Build history of the part. All positions in model axes, mm. A direction names the side the tool comes from. Give positions to 0.01 mm unless a question says otherwise; leave off trailing zeros. Order: outer loops, then holes, each group sorted by start corner. A loop starts at its lowest first (then second) coordinate and runs counter-clockwise, first axis right, second up. Notation, with made-up numbers: M 60.5,1 L 65.5,1 A32 cw 65.5,30 Z; hole C 18.25,52.25 d10. An arc over 180 degrees is marked long. Use CSV: the item, a comma, the result in double quotes. Start each with the question number.
Item 1: Two-plate mould, pull along X, no slides. Class faces 1 (the flat face through (-15, 25.4, -15)), 2 (the cylindrical face through (-26.13, 16.74, -4.58)), 3 (the flat face through (-18, 36.83, -17)): pulls with the +X half, pulls with the -X half, needs draft (parallel to the pull), parting line crosses it, or undercut.
Item 2: Pin check, flat tips, straight feed: P1, Ø4, axis at x = -26.5, y = 17.5, coming from the +Z side; P2, Ø10, axis at x = -8.5, z = -25, coming from the -Y side; P3, Ø4, axis at x = -11.5, y = 37, coming from the +Z side; P4, Ø6.5, axis at x = -17, z = -12, coming from the -Y side. Stop position of each tip, or through.
Item 3: Which spindle directions (+Z, -Z, +X, -X, +Y, -Y) get a long thin tool onto all of the face, cutting with end or side? Do faces 4 (the cylindrical face through (-25.84, 12.52, -12.89)), 5 (the cylindrical face through (-17.343, 40.587, -12.947)), 6 (the cylindrical face through (-4.58, 16.74, -4.35)). Say none if no direction does.
Item 4: Band-saw the part on D-D on x = -16. Write the cut outline in (y, z), plus the area to 3 significant figures.
Item 5: Wall check: line 1 along X through (y, z) = (5, -15); line 2 along Y through (x, z) = (-6.5, -21.5). Give the ranges that are in metal, low to high.
Item 6: Band-saw the part on C-C on z = -6.5. Write the cut outline in (x, y), plus the area to 3 significant figures.
from build123d import *

# Parameters (mm, degrees)
SKETCH3_W           = 30.48
SKETCH3_H           = 30.48
BOSS_EXTRUDE1_DEPTH = 33.02
SKETCH4_R           = 5.08
BOSS_EXTRUDE2_DEPTH = 3.81
SKETCH5_R           = 3.1115
BOSS_EXTRUDE3_DEPTH = 7.62
SKETCH6_R           = 10.8585
CUT_EXTRUDE1_DEPTH  = 25.4
FILLET1_R           = 15.24


with BuildPart() as part:
    # Sketch3 → Boss-Extrude1 (new body)
    with BuildSketch(Plane(origin=(0, 0, 0), x_dir=(1, 0, 0), z_dir=(0, 1, 0))):
        with Locations((-15.24, 15.24)):
            Rectangle(SKETCH3_W, SKETCH3_H)
    extrude(amount=BOSS_EXTRUDE1_DEPTH)

    # Sketch4 → Boss-Extrude2 (add)
    with BuildSketch(Plane(origin=(0, 33.02, 0), x_dir=(1, 0, 0), z_dir=(0, 1, 0))):
        with Locations(Location((-15.24, 15.24, 0), (0, 0, 90))):
            Circle(SKETCH4_R)
    extrude(amount=BOSS_EXTRUDE2_DEPTH)

    # Sketch5 → Boss-Extrude3 (add)
    with BuildSketch(Plane(origin=(0, 36.83, 0), x_dir=(1, 0, 0), z_dir=(0, 1, 0))):
        with Locations(Location((-15.24, 15.24, 0), (0, 0, 90))):
            Circle(SKETCH5_R)
    extrude(amount=BOSS_EXTRUDE3_DEPTH)

    # Sketch6 → Cut-Extrude1 (cut)
    with BuildSketch(Plane.XZ):
        with Locations(Location((-15.24, -15.24, 0), (0, 0, 270))):
            Circle(SKETCH6_R)
    extrude(amount=-CUT_EXTRUDE1_DEPTH, mode=Mode.SUBTRACT)

    # Fillet1
    fillet1_edges = [part.edges().sort_by_distance(p)[0] for p in [
        (-30.48, 16.51, -30.48),
        (0, 16.51, -30.48),
        (-30.48, 16.51, 0),
        (0, 16.51, 0),
    ]]
    fillet(fillet1_edges, radius=FILLET1_R - 0.0001)  # a hair under: the kernel refuses the full size


solid = part.part
Model answer:
1,face 1,"undercut"
1,face 2,"pulls with the -X half"
1,face 3,"needs draft"
2,P1,"stops at z = -3.14"
2,P2,"stops at y = 0"
2,P3,"stops at z = -10.47"
2,P4,"stops at y = 25.4"
3,face 4,"-Y"
3,face 5,"+Y"
3,face 6,"+Z, +X, +Y, -Y"
4,outline,"M 0,-30.46 L 33.02,-30.46 L 33.02,-20.26 L 36.83,-20.26 L 36.83,-18.26 L 44.45,-18.26 L 44.45,-12.22 L 36.83,-12.22 L 36.83,-10.22 L 33.02,-10.22 L 33.02,-0.02 L 0,-0.02 L 0,-4.41 L 25.4,-4.41 L 25.4,-26.07 L 0,-26.07 Z"
4,area,"539 mm^2"
5,line 1,"x = -30.48 to -26.1, -4.38 to 0"
5,line 2,"y = 25.4 to 33.02"
6,outline,"M -27.72,0 L -21.68,0 L -21.68,25.4 L -8.8,25.4 L -8.8,0 L -2.76,0 L -2.76,33.02 L -27.72,33.02 Z"
6,area,"497 mm^2"
